Here's the drawing with two shaded views (mm, measured from the low corner). I have some questions. A direction names the side the tool comes from. Round coordinates to 2 decimals unless told otherwise and drop trailing zeros. Write each loop counter-clockwise with the first axis right and the second up, starting at its lowest first coordinate (ties: lowest second). Pieces come first, ordered by that corner, then holes. Notation, with made-up numbers: (80, 4.5) -> (122, 4.5) arc R32 ccw to (122, 34.5) -> close; hole circle Ø10 at (87.25, -30). An arc over 180 degrees is marked (long way). Use CSV: the item, a comma, the result in double quotes.
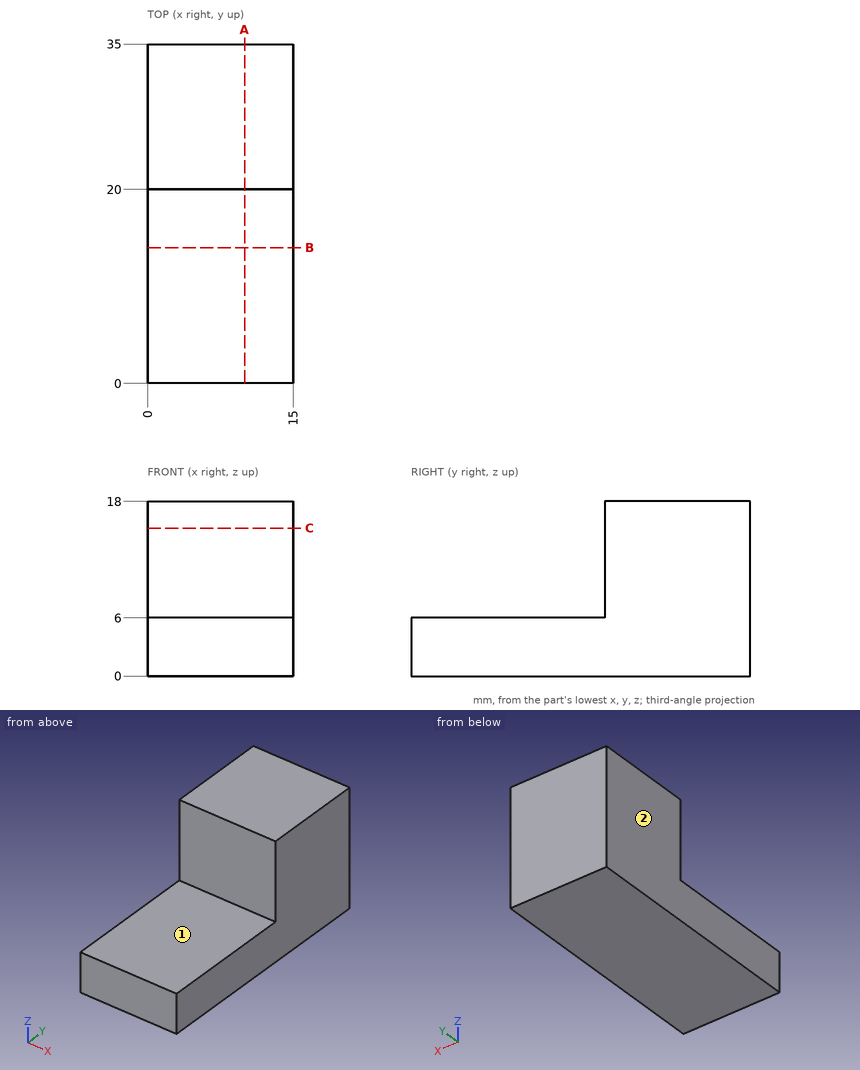
Q1. Suppose I cut it at A-A (x = 10). Write out the boundary of the cut face in (y, z), and give its area (3 significant figures).
Resolved:
outline,"(0, 0) -> (35, 0) -> (35, 18) -> (20, 18) -> (20, 6) -> (0, 6) -> close"
area,"390 mm^2"
Q2. Will these pins go through, and if not, where does the flat tip stop? P1, Ø3, axis at x = 12, z = 9, coming from the -Y side; P2, Ø7.5, axis at x = 9.5, y = 7, coming from the +Z side.
Resolved:
P1,"stops at y = 20"
P2,"stops at z = 6"
Q3. Suppose I cut it at B-B (y = 14). Write out the boundary of the cut face in (x, z), and give its area (3 significant figures).
Resolved:
outline,"(0, 0) -> (15, 0) -> (15, 6) -> (0, 6) -> close"
area,"90.0 mm^2"
Q4. On a 3-axis mill with a long thin cutter (end or side, diameter ignored), from which of +Z, -Z, +X, -X, +Y, -Y can I reach the whole of each face in a straight line? I mean the marked faces 1 and 2. Say none if no direction works.
Resolved:
face 1,"+Z, +X, -X, -Y"
face 2,"+Z, -Z, -X, +Y, -Y"
Q5. Please list where these lines run through material, in increasing order: probe 1 along Z at (x, y) = (4.25, 16); probe 2 along Y at (x, z) = (9, 16).
Resolved:
probe 1,"z = 0 to 6"
probe 2,"y = 20 to 35"
Q6. Suppose I cut it at C-C (z = 15.25). Write out the boundary of the cut face in (x, y).
Resolved:
outline,"(0, 20) -> (15, 20) -> (15, 35) -> (0, 35) -> close"
